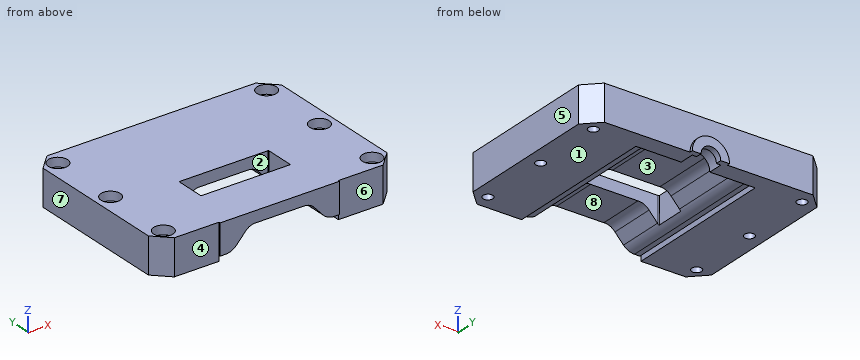
```python
from build123d import *

# Parameters (mm, degrees)
F0_W           = 80
F0_H           = 58
F1_DEPTH       = 6
F3_DEPTH       = 60
F4_SIZE        = 5
F6_D           = 3.3
F6_CBORE_D     = 6.5
F6_CBORE_DEPTH = 3
F8_DEPTH       = 0.5
F10_DEPTH      = 6
F11_R          = 4.8
F12_DEPTH      = 5
F14_DEPTH      = 1
F16_DEPTH      = 12.001


with BuildPart() as f1:
    # F0 (on Top) → F1 (new body, symmetric)
    with BuildSketch(Plane.XY):
        Rectangle(F0_W, F0_H)
    extrude(amount=F1_DEPTH, both=True)

    # F2 (on Front) → F3 (cut, symmetric)
    with BuildSketch(Plane.XZ):
        with BuildLine():
            ThreePointArc((-14.50485, -2.5683595528), (-16.1807477573, -3.7753797852), (-18.2015, -4.2021016015))
            Line((-18.2015, -4.2021016015), (-20, -4.2021016015))
            Line((-20, -4.2021016015), (-20, -6))
            Line((-20, -6), (20, -6))
            Line((20, -6), (20, -4.2021016015))
            Line((20, -4.2021016015), (18.2015, -4.2021016015))
            ThreePointArc((18.2015, -4.2021016015), (16.1807477573, -3.7753797852), (14.50485, -2.5683595528))
            Line((14.50485, -2.5683595528), (11.656, 0.56))
            ThreePointArc((11.656, 0.56), (9.9890562195, 1.8254301669), (7.93, 2.2))
            Line((7.93, 2.2), (-7.93, 2.2))
            ThreePointArc((-7.93, 2.2), (-9.9890562195, 1.8254301669), (-11.656, 0.56))
            Line((-11.656, 0.56), (-14.50485, -2.5683595528))
        make_face()
    extrude(amount=F3_DEPTH, both=True, mode=Mode.SUBTRACT)

    # F4
    f4_edges = [f1.edges().sort_by_distance(p)[0] for p in [
        (-40, 29, 0),
        (-40, -29, 0),
        (40, -29, 0),
        (40, 29, 0),
    ]]
    chamfer(f4_edges, length=F4_SIZE)

    # F6 (through all)
    with Locations(Plane.XY.offset(6)):
        with Locations((-35, 24), (35, 24), (35, 0), (35, -24), (-35, -24), (-35, 0)):
            CounterBoreHole(F6_D / 2, F6_CBORE_D / 2, F6_CBORE_DEPTH)

    # F7 (on face) → F8 (join)
    with BuildSketch(Plane.XZ.offset(29)):
        with BuildLine():
            Line((-20, 6), (-20, -4.2021016015))
            Line((-20, -4.2021016015), (-18.2015, -4.2021016015))
            ThreePointArc((-18.2015, -4.2021016015), (-16.1807477573, -3.7753797852), (-14.50485, -2.5683595528))
            Line((-14.50485, -2.5683595528), (-11.656, 0.56))
            ThreePointArc((-11.656, 0.56), (-9.9890562195, 1.8254301669), (-7.93, 2.2))
            Line((-7.93, 2.2), (7.93, 2.2))
            ThreePointArc((7.93, 2.2), (9.9890562195, 1.8254301669), (11.656, 0.56))
            Line((11.656, 0.56), (14.50485, -2.5683595528))
            ThreePointArc((14.50485, -2.5683595528), (16.1807477573, -3.7753797852), (18.2015, -4.2021016015))
            Line((18.2015, -4.2021016015), (20, -4.2021016015))
            Line((20, -4.2021016015), (20, 6))
            Line((20, 6), (-20, 6))
        make_face()
    extrude(amount=F8_DEPTH)

    # F9 (on face) → F10 (join)
    with BuildSketch(Plane(origin=(0, 29, 0), x_dir=(-1, 0, 0), z_dir=(0, 1, 0))):
        with BuildLine():
            Line((-20, -4.2021016015), (-20, -6))
            Line((-20, -6), (-3.3, -6))
            ThreePointArc((-3.3, -6), (0, -2.7), (3.3, -6))
            Line((3.3, -6), (20, -6))
            Line((20, -6), (20, -4.2021016015))
            Line((20, -4.2021016015), (18.2015, -4.2021016015))
            ThreePointArc((18.2015, -4.2021016015), (16.1807477573, -3.7753797852), (14.50485, -2.5683595528))
            Line((14.50485, -2.5683595528), (11.656, 0.56))
            ThreePointArc((11.656, 0.56), (9.9890562195, 1.8254301669), (7.93, 2.2))
            Line((7.93, 2.2), (-7.93, 2.2))
            ThreePointArc((-7.93, 2.2), (-9.9890562195, 1.8254301669), (-11.656, 0.56))
            Line((-11.656, 0.56), (-14.50485, -2.5683595528))
            ThreePointArc((-14.50485, -2.5683595528), (-16.1807477573, -3.7753797852), (-18.2015, -4.2021016015))
            Line((-18.2015, -4.2021016015), (-20, -4.2021016015))
        make_face()
    extrude(amount=-F10_DEPTH)

    # F11 (on face) → F12 (cut)
    with BuildSketch(Plane.XZ.offset(-23)):
        with Locations((0, -6)):
            Circle(F11_R)
    extrude(amount=-F12_DEPTH, mode=Mode.SUBTRACT)

    # F13 (on face) → F14 (join)
    with BuildSketch(Plane(origin=(0, 29, 0), x_dir=(-1, 0, 0), z_dir=(0, 1, 0))):
        with BuildLine():
            ThreePointArc((-3.3, -6), (0, -2.7), (3.3, -6))
            Line((3.3, -6), (6.25, -6))
            ThreePointArc((6.25, -6), (0, 0.25), (-6.25, -6))
            Line((-6.25, -6), (-3.3, -6))
        make_face()
    extrude(amount=F14_DEPTH)

    # F15 (on face) → F16 (cut, through all)
    with BuildSketch(Plane.XY.offset(6)):
        with BuildLine():
            Line((14.75, -4), (-14.75, -4))
            ThreePointArc((-14.75, -4), (-14.9267766953, -4.0732233047), (-15, -4.25))
            Line((-15, -4.25), (-15, -13.75))
            ThreePointArc((-15, -13.75), (-14.9267766953, -13.9267766953), (-14.75, -14))
            Line((-14.75, -14), (14.75, -14))
            ThreePointArc((14.75, -14), (14.9267766953, -13.9267766953), (15, -13.75))
            Line((15, -13.75), (15, -4.25))
            ThreePointArc((15, -4.25), (14.9267766953, -4.0732233047), (14.75, -4))
        make_face()
    extrude(amount=-F16_DEPTH, mode=Mode.SUBTRACT)


solid = f1.part
```
Read the model definition and answer for the solid it produces. Units are mm, in the model's axes. Face numbers are marked on the shaded views. A direction names the side the tool comes from. Coordinates: 2 decimals unless noted, no trailing zeros. Loops run counter-clockwise (first coordinate to the right, second up) from the corner with the lowest first, then second, coordinate; pieces in that order, holes last. Notation, with made-up numbers: (8.25, 87) -> (55.25, 87) arc R9 cw to (55.25, 92) -> close; hole circle Ø11 at (-12.5, 67). An arc over 180 degrees is marked (long way). Return JSON: item names as keys, results as strings.
Item 1: Flat-ended cylindrical pins translate along their axes: P1, Ø12.5, axis at x = 3.5, y = 8.5, coming from the -Z side; P2, Ø4, axis at x = -22.5, z = 2.5, coming from the -Y side; P3, Ø6, axis at x = 22, z = 1.5, coming from the +Y side. Find the tip coordinate at first contact, or state that the pin passes through.
Answers:
{"P1": "stops at z = 1.92", "P2": "stops at y = -29", "P3": "stops at y = 29"}
Item 2: Find section B-B (x = 0). Determine the outline of the cut face in (y, z), plus the area to 3 significant figures.
Answers:
{"outline": "(-29.5, 2.2) -> (-14, 2.2) -> (-14, 6) -> (-29.5, 6) -> close; (-4, 2.2) -> (23, 2.2) -> (23, -1.2) -> (28, -1.2) -> (28, -2.7) -> (30, -2.7) -> (30, 0.25) -> (29, 0.25) -> (29, 6) -> (-4, 6) -> close", "area": "209 mm2"}
Item 3: Find the intervals of material crossed by probe 1 along Y at (x, z) = (35, 0); probe 2 along X at (y, z) = (-6, 2.75); probe 3 along Y at (x, z) = (-35, 5.1), in increasing order.
Answers:
{"probe 1": "y = -29 to -25.65, -22.35 to -1.65, 1.65 to 22.35, 25.65 to 29", "probe 2": "x = -40 to -15, 15 to 40", "probe 3": "y = -29 to -27.25, -20.75 to -3.25, 3.25 to 20.75, 27.25 to 29"}
Item 4: Find section A-A (y = 0). Count the separate pieces of the cut face and the enclosed holes in it, plus the area to 3 significant figures.
Answers:
{"separate pieces": "3", "enclosed holes": "0", "area": "622 mm2"}
Item 5: For a pull along X with two mould halves and no side action, classify the marked faces 5, 6, 7 and 8 as +X half, -X half, draft (parallel to the pull), parting line (faces both ways), or undercut.
Answers:
{"face 5": "+X half", "face 6": "draft", "face 7": "-X half", "face 8": "undercut"}
Item 6: Find section C-C (x = 21.5). Determine the outline of the cut face in (y, z).
Answers:
{"outline": "(-29, -6) -> (29, -6) -> (29, 6) -> (-29, 6) -> close"}
Item 7: For the marked faces 1, 2, 3 and 4, determine the directions among +Z, -Z, +X, -X, +Y, -Y from which every point of the face is accessible in a straight line to the end or side of a thin tool.
Answers:
{"face 1": "-Z, +X, -X, +Y, -Y", "face 2": "+Z, -Z", "face 3": "-Z, -Y", "face 4": "+Z, -Z, -X, -Y"}
